Source: CAD feature listing. Evaluate the final solid. Frame: model axes, mm. Coordinates: 2 decimals unless noted, no trailing zeros. Order: outer loops, then holes, each group sorted by start corner. A loop starts at its lowest first (then second) coordinate and runs counter-clockwise, first axis right, second up. Notation, with made-up numbers: (14, 80.25) -> (61, 80.25) arc R19 ccw to (61, 92.25) -> close; hole circle Ø9 at (19, 34). An arc over 180 degrees is marked (long way). Write item = value, one per line. Start each with the question number.
Item 1: Section query A-A (z = 257). Output: boundary loops of the cut face in (x, y).
Item 2: Ray query, line 1 along X through (y, z) = (0.25, 173.5); line 2 along Z through (x, y) = (-0.5, -3). Return the intervals inside material, ascending. Write a range as [from, to].
Item 3: Contact query for flat-ended pins moving along their axis: pin 1 (4 mm diameter, centred on y = -3, z = 248.5, fed in from -X); pin 2 (3 mm diameter, centred on y = -2, z = 214, fed in from -X). Output: stop coordinate, or through.
```python
from build123d import *

# Parameters (mm, degrees)
SKETCH1_R           = 4
BOSS_EXTRUDE1_DEPTH = 305
CHAMFER2_SIZE       = 1
CHAMFER3_SIZE       = 1


with BuildPart() as part:
    # Sketch1 → Boss-Extrude1 (new body)
    with BuildSketch(Plane.XY):
        Circle(SKETCH1_R)
    extrude(amount=BOSS_EXTRUDE1_DEPTH)

    # Chamfer2
    chamfer2_edges = [part.edges().sort_by_distance(p)[0] for p in [
        (-4, 0, 0),
    ]]
    chamfer(chamfer2_edges, length=CHAMFER2_SIZE)

    # Chamfer3
    chamfer3_edges = [part.edges().sort_by_distance(p)[0] for p in [
        (-4, 0, 305),
    ]]
    chamfer(chamfer3_edges, length=CHAMFER3_SIZE)


solid = part.part
```
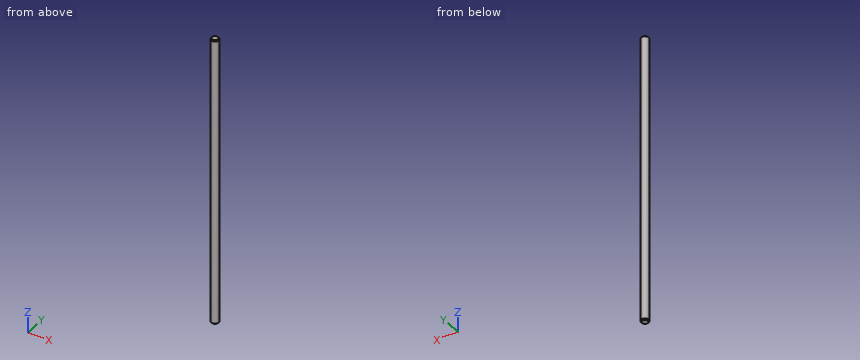
Computed:
q1.outline = circle Ø8 at (0, 0)
q2.line_1 = [-3.99, 3.99]
q2.line_2 = [0.04, 304.96]
q3.pin_1 = -3.87
q3.pin_2 = -3.97
